from build123d import *

# Parameters (mm, degrees)
F2_DEPTH    = 63.5
F3_T1_DEPTH = 154.9490470521


# Not quite as in the source:
# - a fillet or chamfer that OpenCascade refuses, or shapes differently, is made with other operations: its cross-section is extruded or revolved along the edge and cut away or added


with BuildPart() as f2:
    # F1 (on face) → F2 (new body)
    with BuildSketch(Plane.XZ):
        with BuildLine():
            ThreePointArc((-9.525, 0), (0, 9.525), (9.525, 0))
            Line((9.525, 0), (17.9719245062, 0))
            Line((17.9719245062, 0), (31.75, 0))
            Line((31.75, 0), (31.75, 17.5402989774))
            Line((31.75, 17.5402989774), (-31.75, 17.5402989774))
            Line((-31.75, 17.5402989774), (-31.75, 0))
            Line((-31.75, 0), (-17.9475410922, 0))
            Line((-17.9475410922, 0), (-9.525, 0))
        make_face()
    extrude(amount=F2_DEPTH)

    # F3: chamfer of 17.78 on 2 edges, made by hand

    # F3_s2 → F3_t1 (cut)
    with BuildSketch(Plane.XZ.offset(-45.724523526)):
        Polygon((-31.75, 17.78), (-13.97, 0), (-31.75, 0), align=None)
        Polygon((31.75, 17.78), (13.97, 0), (31.75, 0), align=None)
    extrude(amount=F3_T1_DEPTH, mode=Mode.SUBTRACT)


solid = f2.part
Here's how the part is built. I have some questions about the finished solid (model axes, mm). Coordinates: 2 decimals unless noted, no trailing zeros. Loops run counter-clockwise (first coordinate to the right, second up) from the corner with the lowest first, then second, coordinate; pieces in that order, holes last. Notation, with made-up numbers: (44, 19) -> (68, 19) arc R9 ccw to (68, 36) -> close; hole circle Ø3 at (-1.5, 2.25). An arc over 180 degrees is marked (long way). Use one line per item in the form item = value. Start each with the question number.
(1) If we section it at B-B (z = 7.5): Please give me the cut outline in (x, y).
(2) We'd pull the mould along X, two halves only. Please class faces 1 (the face through (22.86, -31.31, 8.89)), 2 (the face through (-22.86, -31.31, 8.89)), 3 (the face through (0, -31, 17.54)), 4 (the face through (-0.209, -31.306, 9.523)): pulls with the +X half, pulls with the -X half, needs draft (parallel to the pull), parting line crosses it, or undercut.
(3) Please list where these lines run through material, in increasing order: line 1 along X through (y, z) = (-5, 5.5); line 2 along X through (y, z) = (-58, 6); line 3 along Z through (x, y) = (19.5, -30).
(4) Will these pins go through, and if not, where does the flat tip stop? pin 1 (1.5 mm diameter, centred on x = 10, z = 2.5, fed in from +Y); pin 2 (10 mm diameter, centred on y = -11, z = 10.5, fed in from -X); pin 3 (4 mm diameter, centred on y = -20.5, z = 4.5, fed in from +X).
(5) If we section it at A-A (y = -43): Please give me the cut outline in (x, z) (3 decimals).
(6) If we section it at D-D (x = -26): Please give me the cut outline in (y, z), then the cut area to 3 significant figures.
(7) If we section it at C-C (x = 27): Please give me the cut outline in (y, z).
Verdict:
q1.outline = (-21.47, -63.5) -> (-5.87, -63.5) -> (-5.87, 0) -> (-21.47, 0) -> close; (5.87, -63.5) -> (21.47, -63.5) -> (21.47, 0) -> (5.87, 0) -> close
q2.face_1 = pulls with the +X half
q2.face_2 = pulls with the -X half
q2.face_3 = needs draft
q2.face_4 = undercut
q3.line_1 = -19.47 to -7.78, 7.78 to 19.47
q3.line_2 = -19.97 to -7.4, 7.4 to 19.97
q3.line_3 = 5.53 to 17.54
q4.pin_1 = 0
q4.pin_2 = -29.47
q4.pin_3 = 20.47
q5.outline = (-31.51, 17.54) -> (-13.97, 0) -> (-9.525, 0) arc R9.525 cw to (9.525, 0) -> (13.97, 0) -> (31.51, 17.54) -> close
q6.outline = (-63.5, 12.03) -> (0, 12.03) -> (0, 17.54) -> (-63.5, 17.54) -> close
q6.area = 350 mm²
q7.outline = (-63.5, 13.03) -> (0, 13.03) -> (0, 17.54) -> (-63.5, 17.54) -> close
